Check sheet for the modelled part. Datum: model origin and axes. Units: mm. A direction names the side the tool comes from. Coordinates: 2 decimals unless noted, no trailing zeros. Order: outer loops, then holes, each group sorted by start corner. A loop starts at its lowest first (then second) coordinate and runs counter-clockwise, first axis right, second up. Notation, with made-up numbers: M 0.5,77.25 L 5.5,77.25 A30 cw 5.5,115.25 Z; hole C -24.75,23 d6. An arc over 180 degrees is marked long. Answer in a Markdown table with one row per item. Add a question column.
Autodesk Fusion 360 part; units mm, degrees
sketch "Sketch1" plane through (0, 0, 0) normal (0, 0, 1) x (1, 0, 0)
  line L0 (20, 15) -> (-20, 15)
  line L1 (-20, 15) -> (-20, -15)
  line L2 (-20, -15) -> (20, -15)
  line L3 (20, -15) -> (20, 15)
  line L4 (20, 15) -> (-20, -15) construction
  line L5 (-20, 15) -> (20, -15) construction
  circle A0 centre (0, 0) radius 11
  circle A1 centre (0, 0) radius 8 construction
  circle A2 centre (0, 0) radius 5
  circle A3 centre (0, 8) radius 1.5
  circle A4 centre (0, -8) radius 1.5
  circle A5 centre (7.9991, -0.1196) radius 1.5
  circle A6 centre (-8, 0) radius 1.5
  line L6 (-20, 15) -> (-17, 15)
  line L7 (-17, 15) -> (-17, -15)
  line L8 (-17, -15) -> (-20, -15)
  line L9 (-20, -15) -> (-20, 15)
  line L10 (-20, 15) -> (-17, -15) construction
  line L11 (-17, 15) -> (-20, -15) construction
  line L12 (0, 15) -> (0, -15) construction
  line L13 (20, -15) -> (20, 15)
  line L14 (17, 15) -> (17, -15)
  line L15 (17, -15) -> (20, -15)
  line L16 (20, 15) -> (17, 15)
  point P0 (-18.5, 0)
  dimension "d1" = 40
  dimension "d2" = 30
  dimension "d3" = 22
  dimension "d4" = 16
  dimension "d5" = 10
  dimension "d6" = 3
  dimension "d7" = 3
  dimension "d9" = 3
  dimension "d10" = 3
  dimension "d11" = 30
  dimension "d12" = 3
extrude "Extrude1" add sketch "Sketch1" along normal blind 3 contours L0 L2 L7 L14
extrude "Extrude2" add sketch "Sketch1" along normal blind 3 contours A0
extrude "Extrude3" add sketch "Sketch1" against normal blind 3 contours A0
extrude "Extrude4" add sketch "Sketch1" along normal blind 17 contours L0 L1 L2 L6 L7 L8 L9
extrude "Extrude5" add sketch "Sketch1" along normal blind 17 contours L0 L2 L3 L13 L14 L15 L16
sketch "Sketch2" plane through (0, 0, 0) normal (1, 0, 0) x (0, 1, 0)
  line L0 (-15, 12.9476) -> (15, 12.9476) construction
  line L1 (-15, 16.9476) -> (15, 16.9476) construction
  line L2 (0, 16.9476) -> (0, 0) construction
  line L3 (-11, 16.9476) -> (-11, 0) construction
  line L4 (11, 16.9476) -> (11, 0) construction
  circle A0 centre (-11, 12.9476) radius 1.6
  circle A1 centre (11, 12.9476) radius 1.6
  dimension "d23" = 4
  dimension "d24" = 11
  dimension "d25" = 3.2
extrude "Extrude6" cut sketch "Sketch2" along normal blind 28
extrude "Extrude7" cut sketch "Sketch2" against normal blind 25
1. Go/stop test with flat-tipped pins: pin 1 Ø8 at (x, y) = (-5, 9) entering from +Z; pin 2 Ø2 at (x, y) = (13.5, -4) entering from -Z. Record where each tip stops, or that it passes through.
2. Section check C-C on y = 8. Enter the section's corners in (x, z).
3. Section check A-A on x = 0. Enter the section's corners in (y, z).
4. Section check B-B on z = 15.75. Enter the section's corners in (x, y).
5. Scan lines: line 1 (X direction, y = 0.75, z = 7); line 2 (Y direction, x = 0, z = -1.4); line 3 (Z direction, x = -17.9, y = -11). Record each from-to range of solid material in increasing order.
6. Release check for a two-part mould opening along Z. For faces 4 (the flat face through (-19, 0, 17)), 5 (the flat face through (-0.3, -15, 2.7)), 6 (the cylindrical face through (-18.48, 9.82, 14.03)) record: released by +Z, released by -Z, zero draft, split by the parting line, or undercut.
7. Set-up check for faces 1 (the flat face through (17, 0, 10)), 2 (the flat face through (-5, 10, 0)), 3 (the cylindrical face through (-1.08, 4.88, -0.04)): record each of +Z, -Z, +X, -X, +Y, -Y from which the full face is reachable in a straight line by a thin tool's end or side.
8. Section check D-D on x = 4. Enter the section's corners in (y, z).
Result sheet:
| question | item | result |
|---|---|---|
| 1 | pin 1 | z = 3 |
| 1 | pin 2 | z = 0 |
| 2 | outline | M -20,0 L -7.55,0 L -7.55,-3 L -1.5,-3 L -1.5,3 L -17,3 L -17,17 L -20,17 Z; M 1.5,-3 L 7.55,-3 L 7.55,0 L 20,0 L 20,17 L 17,17 L 17,3 L 1.5,3 Z |
| 3 | outline | M -15,0 L -11,0 L -11,-3 L -9.5,-3 L -9.5,3 L -15,3 Z; M -6.5,-3 L -5,-3 L -5,3 L -6.5,3 Z; M 5,-3 L 6.5,-3 L 6.5,3 L 5,3 Z; M 9.5,-3 L 11,-3 L 11,0 L 15,0 L 15,3 L 9.5,3 Z |
| 4 | outline | M -20,-15 L -17,-15 L -17,15 L -20,15 Z; M 17,-15 L 20,-15 L 20,15 L 17,15 Z |
| 5 | line 1 | -20 to -17, 17 to 20 |
| 5 | line 2 | -11 to -9.5, -6.5 to -5, 5 to 6.5, 9.5 to 11 |
| 5 | line 3 | 0 to 11.35, 14.55 to 17 |
| 6 | face 4 | released by +Z |
| 6 | face 5 | zero draft |
| 6 | face 6 | undercut |
| 7 | face 1 | +Z, +Y, -Y |
| 7 | face 2 | -Z |
| 7 | face 3 | +Z, -Z |
| 8 | outline | M -15,0 L -10.25,0 L -10.25,-3 L -3,-3 L -3,3 L -15,3 Z; M 3,-3 L 10.25,-3 L 10.25,0 L 15,0 L 15,3 L 3,3 Z |
